The model under review builds one solid part; all positions refer to its coordinate system, in mm. Face numbers are marked on the shaded views. Give positions to 0.01 mm unless a question says otherwise; leave off trailing zeros. Loops run counter-clockwise (first coordinate to the right, second up) from the corner with the lowest first, then second, coordinate; pieces in that order, holes last. Notation, with made-up numbers: (-7.75, 54) - (-3.75, 54) arc R13 ccw to (-3.75, 60) - close; hole circle Ø2 at (54.25, 24.25). An arc over 180 degrees is marked (long way). Answer as a JSON object with one key per item and string values.
from build123d import *

# Parameters (mm, degrees)
F0_W     = 1000
F0_H     = 800
F1_DEPTH = 15
F3_D     = 50
F4_D     = 20
F5_D     = 17.5
F6_R     = 20
F7_SIZE  = 50


with BuildPart() as f1:
    # F0 (on Front) → F1 (new body, symmetric)
    with BuildSketch(Plane.XZ):
        Rectangle(F0_W, F0_H)
    extrude(amount=F1_DEPTH, both=True)

    # F3 (through all)
    with Locations(Plane.XZ.offset(15)):
        with Locations((-200, 200)):
            Hole(F3_D / 2)

    # F4 (through all)
    with Locations(Plane.XZ.offset(15)):
        with Locations((-150, -200)):
            Hole(F4_D / 2)

    # F5 (through all)
    with Locations(Plane.XZ.offset(15)):
        with Locations((320, 200)):
            Hole(F5_D / 2)

    # F6
    f6_edges = [f1.edges().sort_by_distance(p)[0] for p in [
        (-500, 0, 400),
    ]]
    fillet(f6_edges, radius=F6_R)

    # F7
    f7_edges = [f1.edges().sort_by_distance(p)[0] for p in [
        (-500, 0, -400),
    ]]
    chamfer(f7_edges, length=F7_SIZE)


solid = f1.part
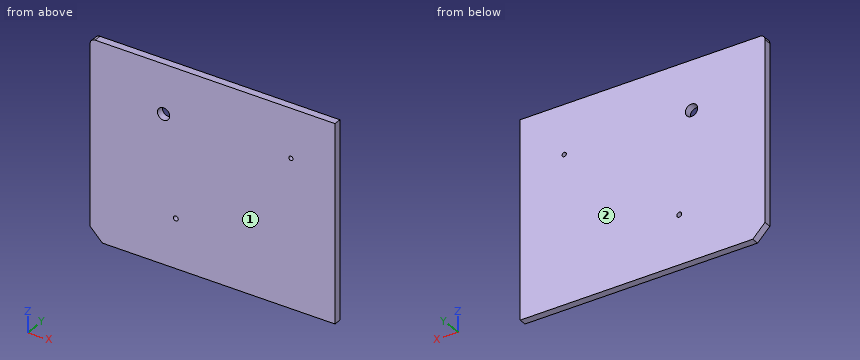
Q1. Clearance check with a flat-ended pin moving along its axis: pin 1 Ø16 at (x, z) = (320, 200) entering from -Y. State where the tip first meets the part, or that it passes through.
Results:
{"pin 1": "passes through"}
Q2. The part is to be moulded in two halves that separate along Y. For the marked faces 1 and 2, say which applies: +Y half, -Y half, draft (parallel to the pull), parting line (faces both ways), or undercut.
Results:
{"face 1": "-Y half", "face 2": "+Y half"}
Q3. Consider section A-A, the plane x = -200. State the section outline as (y, z) points.
Results:
{"outline": "(-15, -400) - (15, -400) - (15, 175) - (-15, 175) - close; (-15, 225) - (15, 225) - (15, 400) - (-15, 400) - close"}
Q4. To check wall thickness, follow probe 1 along Z at (x, y) = (320, 0.75); probe 2 along Z at (x, y) = (-150, 6.75); probe 3 along X at (y, z) = (2.5, -200.5). State the ranges of each line that lie inside material, in increasing order. Write a range as [from, to].
Results:
{"probe 1": "z = [-400, 191.25], [208.75, 400]", "probe 2": "z = [-400, -210], [-190, 400]", "probe 3": "x = [-500, -159.99], [-140.01, 500]"}
